```python
from build123d import *

# Parameters (mm, degrees)
SKETCH1_W            = 40.64
SKETCH1_H            = 33.02
BOSS_EXTRUDE1_DEPTH  = 25.4
SKETCH2_W            = 7.62
SKETCH2_H            = 7.62
CUT_EXTRUDE1_DEPTH   = 26.4
SKETCH3_W            = 7.62
SKETCH3_H            = 7.62
CUT_EXTRUDE2_DEPTH   = 26.4
SKETCH4_R            = 12.446
BOSS_EXTRUDE2_DEPTH  = 2.54
SKETCH5_R            = 12.446
BOSS_EXTRUDE3_DEPTH  = 2.794
BOSS_EXTRUDE3_TAPER  = -45
SKETCH6_R            = 15.24
BOSS_EXTRUDE4_DEPTH  = 13.97
SKETCH7_R            = 12.446
BOSS_EXTRUDE5_DEPTH  = 2.54
SKETCH8_R            = 12.446
BOSS_EXTRUDE6_DEPTH  = 2.794
BOSS_EXTRUDE6_TAPER  = -45
SKETCH9_R            = 15.24
BOSS_EXTRUDE7_DEPTH  = 13.97
SKETCH10_R           = 12.446
BOSS_EXTRUDE8_DEPTH  = 2.54
SKETCH11_R           = 12.446
BOSS_EXTRUDE9_DEPTH  = 2.794
BOSS_EXTRUDE9_TAPER  = -45
SKETCH12_R           = 15.24
BOSS_EXTRUDE10_DEPTH = 13.97
SKETCH13_R           = 9.271
CUT_EXTRUDE3_DEPTH   = 52.10556
CUT_EXTRUDE4_REACH   = 43.293
SKETCH14_R           = 9.271
SKETCH15_R           = 10.611739
CUT_EXTRUDE5_DEPTH   = 1.451356
CUT_EXTRUDE5_TAPER   = 45
SKETCH16_R           = 8.849363403
CUT_EXTRUDE6_DEPTH   = 12.119864
CUT_EXTRUDE6_TAPER   = -1.47
SKETCH17_R           = 10.611739
CUT_EXTRUDE7_DEPTH   = 1.451356
CUT_EXTRUDE7_TAPER   = 45
SKETCH18_R           = 8.849363403
CUT_EXTRUDE8_DEPTH   = 12.119864
CUT_EXTRUDE8_TAPER   = -1.47
SKETCH21_R           = 8.849363403
CUT_EXTRUDE9_DEPTH   = 12.119864
CUT_EXTRUDE9_TAPER   = -1.47
CHAMFER1_SIZE        = 1.016
CHAMFER2_SIZE        = 1.016
CHAMFER3_SIZE        = 1.016


with BuildPart() as part:
    # Sketch1 → Boss-Extrude1 (new body)
    with BuildSketch(Plane(origin=(0, 12.7, 0), x_dir=(-1, 0, 0), z_dir=(0, 1, 0))):
        with Locations((-39.624, -3.81)):
            Rectangle(SKETCH1_W, SKETCH1_H)
    extrude(amount=-BOSS_EXTRUDE1_DEPTH)

    # Sketch2 → Cut-Extrude1 (cut, through all)
    with BuildSketch(Plane.XZ.offset(12.7)):
        with Locations((56.134, -16.51)):
            Rectangle(SKETCH2_W, SKETCH2_H)
    extrude(amount=-CUT_EXTRUDE1_DEPTH, mode=Mode.SUBTRACT)

    # Sketch3 → Cut-Extrude2 (cut, through all)
    with BuildSketch(Plane.XZ.offset(12.7)):
        with Locations((23.114, -16.51)):
            Rectangle(SKETCH3_W, SKETCH3_H)
    extrude(amount=-CUT_EXTRUDE2_DEPTH, mode=Mode.SUBTRACT)

    # Sketch4 → Boss-Extrude2 (add)
    with BuildSketch(Plane.ZY.offset(-19.304)):
        Circle(SKETCH4_R)
    extrude(amount=BOSS_EXTRUDE2_DEPTH)

    # Sketch5 → Boss-Extrude3 (add)
    with BuildSketch(Plane.ZY.offset(-16.764)):
        Circle(SKETCH5_R)
    extrude(amount=BOSS_EXTRUDE3_DEPTH, taper=BOSS_EXTRUDE3_TAPER)

    # Sketch6 → Boss-Extrude4 (add)
    with BuildSketch(Plane.ZY.offset(-13.97)):
        Circle(SKETCH6_R)
    extrude(amount=BOSS_EXTRUDE4_DEPTH)

    # Sketch7 → Boss-Extrude5 (add)
    with BuildSketch(Plane(origin=(59.944, 0, 0), x_dir=(0, 0, -1), z_dir=(1, 0, 0))):
        Circle(SKETCH7_R)
    extrude(amount=BOSS_EXTRUDE5_DEPTH)

    # Sketch8 → Boss-Extrude6 (add)
    with BuildSketch(Plane(origin=(62.484, 0, 0), x_dir=(0, 0, -1), z_dir=(1, 0, 0))):
        Circle(SKETCH8_R)
    extrude(amount=BOSS_EXTRUDE6_DEPTH, taper=BOSS_EXTRUDE6_TAPER)

    # Sketch9 → Boss-Extrude7 (add)
    with BuildSketch(Plane(origin=(65.278, 0, 0), x_dir=(0, 0, -1), z_dir=(1, 0, 0))):
        Circle(SKETCH9_R)
    extrude(amount=BOSS_EXTRUDE7_DEPTH)

    # Sketch10 → Boss-Extrude8 (add)
    with BuildSketch(Plane(origin=(0, 0, -20.32), x_dir=(-1, 0, 0), z_dir=(0, 0, -1))):
        with Locations((-39.624, 0)):
            Circle(SKETCH10_R)
    extrude(amount=BOSS_EXTRUDE8_DEPTH)

    # Sketch11 → Boss-Extrude9 (add)
    with BuildSketch(Plane(origin=(0, 0, -22.86), x_dir=(-1, 0, 0), z_dir=(0, 0, -1))):
        with Locations((-39.624, 0)):
            Circle(SKETCH11_R)
    extrude(amount=BOSS_EXTRUDE9_DEPTH, taper=BOSS_EXTRUDE9_TAPER)

    # Sketch12 → Boss-Extrude10 (add)
    with BuildSketch(Plane(origin=(0, 0, -25.654), x_dir=(-1, 0, 0), z_dir=(0, 0, -1))):
        with Locations((-39.624, 0)):
            Circle(SKETCH12_R)
    extrude(amount=BOSS_EXTRUDE10_DEPTH)

    # Sketch13 → Cut-Extrude3 (cut)
    with BuildSketch(Plane(origin=(13.57122, 0, 0), x_dir=(0, -1, 0), z_dir=(-1, 0, 0))):
        Circle(SKETCH13_R)
    extrude(amount=-CUT_EXTRUDE3_DEPTH, mode=Mode.SUBTRACT)

    # Sketch14 → Cut-Extrude4 (cut, up to next)
    with BuildSketch(Plane(origin=(0, 0, -26.05278), x_dir=(-1, 0, 0), z_dir=(0, 0, -1)), mode=Mode.PRIVATE) as cut_extrude4_sk1:
        with Locations((-39.624, 0)):
            Circle(SKETCH14_R)
    cut_extrude4_tool1 = extrude(cut_extrude4_sk1.sketch, amount=-CUT_EXTRUDE4_REACH, mode=Mode.PRIVATE) & part.part
    add(cut_extrude4_tool1.solids().sort_by_distance((39.624, 0, -26.05278))[0], mode=Mode.SUBTRACT)

    # Sketch15 → Cut-Extrude5 (cut)
    with BuildSketch(Plane(origin=(0, 0, -39.624), x_dir=(-1, 0, 0), z_dir=(0, 0, -1))):
        with Locations((-39.624, 0)):
            Circle(SKETCH15_R)
    extrude(amount=-CUT_EXTRUDE5_DEPTH, taper=CUT_EXTRUDE5_TAPER, mode=Mode.SUBTRACT)

    # Sketch16 → Cut-Extrude6 (cut)
    with BuildSketch(Plane.XY.offset(-26.05278)):
        with Locations((39.624, 0)):
            Circle(SKETCH16_R)
    extrude(amount=-CUT_EXTRUDE6_DEPTH, taper=CUT_EXTRUDE6_TAPER, mode=Mode.SUBTRACT)

    # Sketch17 → Cut-Extrude7 (cut)
    with BuildSketch(Plane.ZY):
        Circle(SKETCH17_R)
    extrude(amount=-CUT_EXTRUDE7_DEPTH, taper=CUT_EXTRUDE7_TAPER, mode=Mode.SUBTRACT)

    # Sketch18 → Cut-Extrude8 (cut)
    with BuildSketch(Plane(origin=(13.57122, 0, 0), x_dir=(0, 0, -1), z_dir=(1, 0, 0))):
        Circle(SKETCH18_R)
    extrude(amount=-CUT_EXTRUDE8_DEPTH, taper=CUT_EXTRUDE8_TAPER, mode=Mode.SUBTRACT)

    # Sketch19 → Hole1 (revolve, cut)
    with BuildSketch(Plane(origin=(79.248, 0, 0), x_dir=(0, 0, -1), z_dir=(0, 1, 0))):
        Polygon((0, 0), (0, 1.451356), (10.611739, 1.451356), (9.160383, 0), align=None)
    revolve(axis=Axis((-30.752, 0, 0), (1, 0, 0)), mode=Mode.SUBTRACT)

    # Sketch21 → Cut-Extrude9 (cut)
    with BuildSketch(Plane.ZY.offset(-65.67678)):
        Circle(SKETCH21_R)
    extrude(amount=-CUT_EXTRUDE9_DEPTH, taper=CUT_EXTRUDE9_TAPER, mode=Mode.SUBTRACT)

    # Chamfer1
    chamfer1_edges = [part.edges().sort_by_distance(p)[0] for p in [
        (0, 0, -15.24),
    ]]
    chamfer(chamfer1_edges, length=CHAMFER1_SIZE)

    # Chamfer2
    chamfer2_edges = [part.edges().sort_by_distance(p)[0] for p in [
        (79.248, 0, 15.24),
    ]]
    chamfer(chamfer2_edges, length=CHAMFER2_SIZE)

    # Chamfer3
    chamfer3_edges = [part.edges().sort_by_distance(p)[0] for p in [
        (54.864, 0, -39.624),
    ]]
    chamfer(chamfer3_edges, length=CHAMFER3_SIZE)


solid = part.part
```
Geometry check sheet. Reference: the model listing, model coordinates, mm. A direction names the side the tool comes from. Give positions to 0.01 mm unless a question says otherwise; leave off trailing zeros. Order: outer loops, then holes, each group sorted by start corner. A loop starts at its lowest first (then second) coordinate and runs counter-clockwise, first axis right, second up. Notation, with made-up numbers: (10, 27.25) - (62, 27.25) arc R6 ccw to (62, 36.25) - close; hole circle Ø1 at (83.25, -11). An arc over 180 degrees is marked (long way). Answer in a Markdown table with one row per item. Add a question column.
Q1. Gauge pin test, flat ends, axial feed: pin 1 (4 mm diameter, centred on x = 71, y = -11.5, fed in from +Z); pin 2 (12 mm diameter, centred on x = 47.5, z = -29.5, fed in from +Y); pin 3 (1.5 mm diameter, centred on x = 65.5, z = -5, fed in from +Y). Record the tip position at first contact, or that the pin passes through.
Q2. Mould release check, pull along Y, two halves, no side actions. Record for faces 5 (the flat face through (79.248, -9, -3)), 6 (the cylindrical face through (7.58, -14.88, -3.3)), 7 (the flat face through (32, -5, -26.053)): pulls with the +Y half, pulls with the -Y half, needs draft (parallel to the pull), parting line crosses it, or undercut.
Q3. Tool access check on faces 1 (the flat face through (23, 0, -12.7)), 2 (the conical face through (30.626, 0.396, -32.198)), 3 (the flat face through (59.944, -12, -4)), 4 (the conical face through (71.82, 8.93, -1.17)). Record the directions out of +Z, -Z, +X, -X, +Y, -Y that give a thin tool (end or side, any length) a straight path to the whole face; none if there is none.
Q4. Cross-section at C-C, the plane y = 6. Count the separate pieces of the cut face and the enclosed holes in it, then the cut area to 3 significant figures.
Q5. Cross-section at A-A, the plane x = 22.5. Enter the section's corners in (y, z), then the cut area to 3 significant figures.
Q6. Material ranges on probe 1 along Z at (x, y) = (28, 0); probe 2 along X at (y, z) = (10.5, -10); probe 3 along Z at (x, y) = (75, 1.5), recorded low to high. Write a range as from..to.
Q7. Cross-section at D-D, the plane z = -22. Enter the section's corners in (x, y).
Q8. Cross-section at B-B, the plane z = -27.5. Enter the section's corners in (x, y), then the cut area to 3 significant figures.
Check values:
| question | item | result |
|---|---|---|
| 1 | pin 1 | stops at z = 11.92 |
| 1 | pin 2 | stops at y = 15.12 |
| 1 | pin 3 | stops at y = 14.64 |
| 2 | face 5 | needs draft |
| 2 | face 6 | parting line crosses it |
| 2 | face 7 | undercut |
| 3 | face 1 | +Y, -Y |
| 3 | face 2 | -Z |
| 3 | face 3 | none |
| 3 | face 4 | +X |
| 4 | separate pieces | 3 |
| 4 | enclosed holes | 0 |
| 4 | area | 1,210 mm^2 |
| 5 | outline | (-12.7, -12.7) - (12.7, -12.7) - (12.7, 12.7) - (-12.7, 12.7) - close; hole circle Ø18.54 at (0, 0) |
| 5 | area | 375 mm^2 |
| 6 | probe 1 | z = -39.62..-9.27, 9.27..12.7 |
| 6 | probe 2 | x = 0.28..14.71, 19.3..59.94, 64.54..78.97 |
| 6 | probe 3 | z = -15.17..-8.96, 8.96..15.17 |
| 7 | outline | circle Ø24.89 at (39.62, 0); hole circle Ø18.54 at (39.62, 0) |
| 8 | outline | circle Ø30.48 at (39.62, 0); hole circle Ø17.77 at (39.62, 0) |
| 8 | area | 482 mm^2 |
